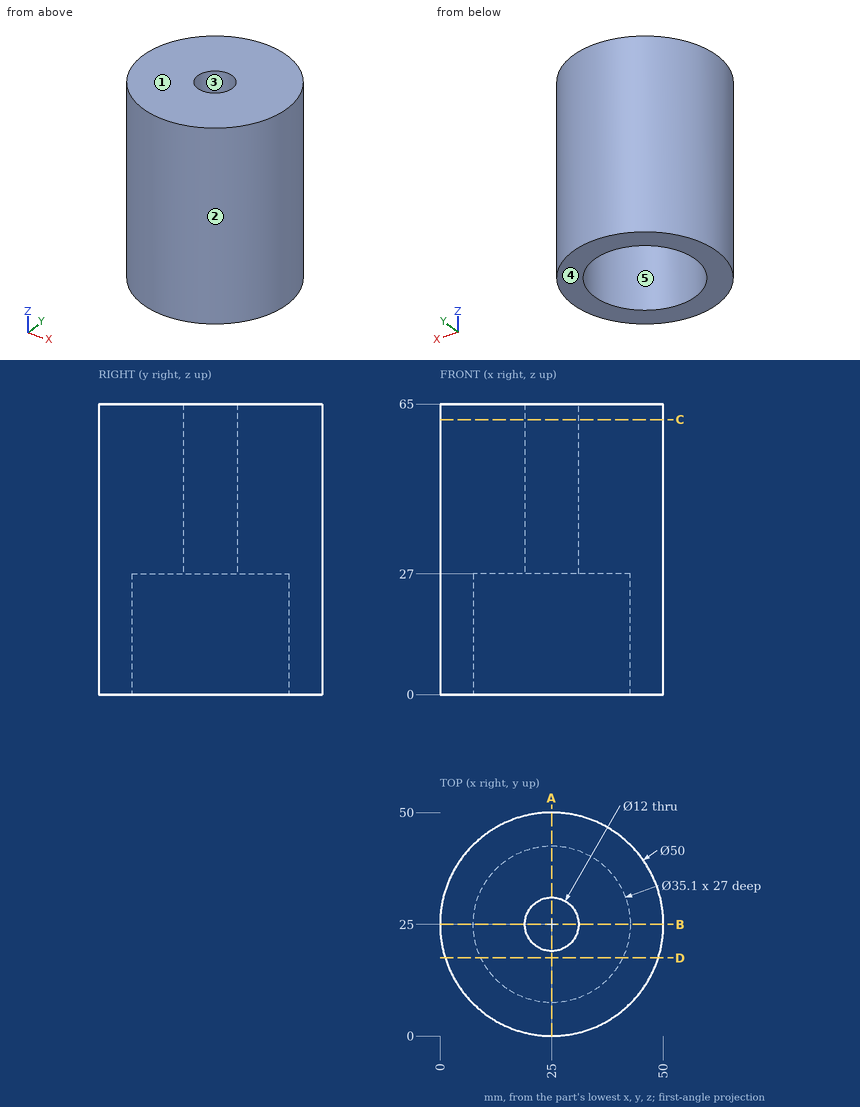
Here's the drawing with two shaded views (mm, measured from the low corner). I have some questions. A direction names the side the tool comes from. Coordinates: 2 decimals unless noted, no trailing zeros. Order: outer loops, then holes, each group sorted by start corner. A loop starts at its lowest first (then second) coordinate and runs counter-clockwise, first axis right, second up. Notation, with made-up numbers: M 58,21 L 80,21 A12 cw 80,32 Z; hole C 31.25,-16 d9. An arc over 180 degrees is marked long. Answer as CSV lines item,"result".
Item 1: On a 3-axis mill with a long thin cutter (end or side, diameter ignored), from which of +Z, -Z, +X, -X, +Y, -Y can I reach the whole of each face in a straight line? I mean the marked faces 4 and 5. Say none if no direction works.
Results found:
face 4,"-Z, +X, -X, +Y, -Y"
face 5,"-Z"
Item 2: We'd pull the mould along Y, two halves only. Please class the marked faces 1, 2 and 3: +Y half, -Y half, draft (parallel to the pull), parting line (faces both ways), or undercut.
Results found:
face 1,"draft"
face 2,"parting line"
face 3,"undercut"
Item 3: Imagine slicing it at C-C on z = 61.5. Write out the boundary of the cut face in (x, y).
Results found:
outline,"C 25,25 d50; hole C 25,25 d12"
Item 4: If I drill on line 1 (Y direction, x = 25, z = 44); line 2 (Y direction, x = 25, z = 12); line 3 (Z direction, x = 15.5, y = 38), over which ranges is the centre line in solid material (lowest first)?
Results found:
line 1,"0 to 19, 31 to 50"
line 2,"0 to 7.45, 42.55 to 50"
line 3,"27 to 65"
Item 5: For pin 1 (1 mm diameter, centred on x = 33, y = 10, fed in from -Z); pin 2 (10 mm diameter, centred on x = 43, z = 18, fed in from -Y); pin 3 (1 mm diameter, centred on x = 19, z = 38.5, fed in from -Y), each with a flat end and sliding along its axis, tell me the tip position at first contact or that it passes through.
Results found:
pin 1,"z = 27"
pin 2,"y = 3.65"
pin 3,"y = 0.61"
Item 6: Imagine slicing it at A-A on x = 25. Write out the boundary of the cut face in (y, z), plus the area to 3 significant figures.
Results found:
outline,"M 0,0 L 7.45,0 L 7.45,27 L 19,27 L 19,65 L 0,65 Z; M 31,27 L 42.55,27 L 42.55,0 L 50,0 L 50,65 L 31,65 Z"
area,"1,850 mm2"
Item 7: Imagine slicing it at D-D on y = 17.5. Write out the boundary of the cut face in (x, z), plus the area to 3 significant figures.
Results found:
outline,"M 1.15,0 L 9.13,0 L 9.13,27 L 40.87,27 L 40.87,0 L 48.85,0 L 48.85,65 L 1.15,65 Z"
area,"2,240 mm2"
